from build123d import *

# Parameters (mm, degrees)
REDONDEO1_R             = 1
CHAFL_N1_SIZE           = 1
CROQUIS2_R              = 2
SALIENTE_EXTRUIR1_DEPTH = 3


with BuildPart() as part:
    # Croquis1 → Revolución1 (revolve)
    with BuildSketch(Plane.XY):
        Polygon((-16, 0), (-16, 4.5), (0, 4.5), (0, 7.5), (10, 7.5), (10, 3), (20, 3), (20, 0), align=None)
    revolve(axis=Axis((-18.371134021, 0, 0), (1, 0, 0)))

    # Redondeo1
    redondeo1_edges = [part.edges().sort_by_distance(p)[0] for p in [
        (0, -4.5, 0),
    ]]
    fillet(redondeo1_edges, radius=REDONDEO1_R)

    # Chaflán1
    chafl_n1_edges = [part.edges().sort_by_distance(p)[0] for p in [
        (-16, -4.5, 0),
    ]]
    chamfer(chafl_n1_edges, length=CHAFL_N1_SIZE)

    # Croquis2 → Saliente-Extruir1 (add)
    with BuildSketch(Plane(origin=(10, 0, 0), x_dir=(0, 0, -1), z_dir=(1, 0, 0))):
        with BuildLine():
            Line((-11, -15), (11, -15))
            ThreePointArc((11, -15), (13.828427125, -13.828427125), (15, -11))
            Line((15, -11), (15, 11))
            ThreePointArc((15, 11), (13.828427125, 13.828427125), (11, 15))
            Line((11, 15), (-11, 15))
            ThreePointArc((-11, 15), (-13.828427125, 13.828427125), (-15, 11))
            Line((-15, 11), (-15, -11))
            ThreePointArc((-15, -11), (-13.828427125, -13.828427125), (-11, -15))
        make_face()
        with Locations((-10, 10)):
            Circle(CROQUIS2_R, mode=Mode.SUBTRACT)
        with Locations((10, 10)):
            Circle(CROQUIS2_R, mode=Mode.SUBTRACT)
        with Locations((10, -10)):
            Circle(CROQUIS2_R, mode=Mode.SUBTRACT)
        with Locations((-10, -10)):
            Circle(CROQUIS2_R, mode=Mode.SUBTRACT)
    extrude(amount=SALIENTE_EXTRUIR1_DEPTH)


solid = part.part
CAD build for the part. Positions are in the model's coordinates, mm. A direction names the side the tool comes from. Round coordinates to 2 decimals unless told otherwise and drop trailing zeros. Loops run counter-clockwise (first coordinate to the right, second up) from the corner with the lowest first, then second, coordinate; pieces in that order, holes last. Notation, with made-up numbers: M 12.25,36.25 L 21.25,36.25 A21 ccw 21.25,74.25 Z; hole C 0,12 d7. An arc over 180 degrees is marked long. One line per question, with ' | ' between items. Start each with the question number.
Item 1: Pin check, flat tips, straight feed: pin 1 Ø6.5 at (y, z) = (10, -10) entering from +X; pin 2 Ø6.5 at (y, z) = (-10, -10) entering from -X; pin 3 Ø10 at (x, y) = (4.5, 0.5) entering from -Z. Stop position of each tip, or through.
Item 2: Which spindle directions (+Z, -Z, +X, -X, +Y, -Y) get a long thin tool onto all of the face, cutting with end or side? Do faces 1 (the cylindrical face through (17, -3, 0)), 2 (the cylindrical face through (11.479, 13.797, -13.859)), 3 (the flat face through (0, 4, 4)). Say none if no direction does.
Item 3: Wall check: line 1 (Y direction, x = 11.7, z = -10); line 2 (X direction, y = -10.25, z = -3); line 3 (X direction, y = -3, z = -5.5). Give the ranges that are in metal, low to high.
Item 4: Cut at A-A, the plane x = 12. Write the cut outline in (y, z), plus the area to 3 significant figures.
Item 5: Cut at D-D, the plane y = 0. Write the cut outline in (x, z).
Item 6: Two-plate mould, pull along Z, no slides. Class faces 4 (the cylindrical face through (-7.9, -0.59, 4.46)), 5 (the cylindrical face through (11, -8, -10)), 6 (the cylindrical face through (11, 12, 10)), 7 (the flat face through (11, 0, 15)): pulls with the +Z half, pulls with the -Z half, needs draft (parallel to the pull), parting line crosses it, or undercut.
Item 7: Cut at B-B, the plane z = -10. Write the cut outline in (x, y).
Responses:
1) pin 1: stops at x = 13 | pin 2: stops at x = 10 | pin 3: stops at z = -7.5
2) face 1: +X | face 2: -Z, +X, -X, +Y | face 3: -X
3) line 1: y = -15 to -12, -8 to 8, 12 to 15 | line 2: x = 10 to 13 | line 3: x = 0 to 13
4) outline: M -15,-11 A4 ccw -11,-15 L 11,-15 A4 ccw 15,-11 L 15,11 A4 ccw 11,15 L -11,15 A4 ccw -15,11 Z; hole C -10,-10 d4; hole C -10,10 d4; hole C 10,-10 d4; hole C 10,10 d4 | area: 836 mm²
5) outline: M -16,-3.5 L -15,-4.5 L -1,-4.5 A1 cw 0,-5.5 L 0,-7.5 L 10,-7.5 L 10,-15 L 13,-15 L 13,-3 L 20,-3 L 20,3 L 13,3 L 13,15 L 10,15 L 10,7.5 L 0,7.5 L 0,5.5 A1 cw -1,4.5 L -15,4.5 L -16,3.5 Z
6) face 4: parting line crosses it | face 5: undercut | face 6: undercut | face 7: pulls with the +Z half
7) outline: M 10,-15 L 13,-15 L 13,-12 L 10,-12 Z; M 10,-8 L 13,-8 L 13,8 L 10,8 Z; M 10,12 L 13,12 L 13,15 L 10,15 Z
